Read the model definition and answer for the solid it produces. Units are mm, in the model's axes. Coordinates: 2 decimals unless noted, no trailing zeros. Write each loop counter-clockwise with the first axis right and the second up, starting at its lowest first coordinate (ties: lowest second). Pieces come first, ordered by that corner, then holes. Notation, with made-up numbers: (23.25, 56.5) -> (44.25, 56.5) arc R17 ccw to (44.25, 65.5) -> close; hole circle Ø7 at (46, -25.75). An arc over 180 degrees is marked (long way). Use CSV: the item, a comma, the result in double quotes.
Autodesk Inventor part; units mm, degrees
ref_plane "YZ Plane" through (0, 0, 0) normal (1, 0, 0) x (0, 1, 0)
ref_plane "XZ Plane" through (0, 0, 0) normal (0, 1, 0) x (-1, 0, 0)
ref_plane "XY Plane" through (0, 0, 0) normal (0, 0, 1) x (1, 0, 0)
sketch "Sketch1" plane through (0, 0, 0) normal (0, 0, 1) x (1, 0, 0)
  line L0 (0, 0) -> (5.08, 0)
  line L1 (5.08, 0) -> (5.08, 7.62)
  line L2 (0, 7.62) -> (0, 0)
  arc A0 (5.08, 7.62) -> (0, 7.62) centre (2.54, 7.62) ccw
  dimension "d0" = 5.08
  dimension "d1" = 7.62
extrude "Extrusion1" add sketch "Sketch1" along normal blind 19.05
sketch "Sketch2" plane through (5.08, 0, 0) normal (1, 0, 0) x (0, 0, -1)
  line L0 (-19.05, 7.62) -> (-19.05, 0)
  line L1 (0, 0) -> (0, 7.62)
  line L2 (0, 7.62) -> (-19.05, 7.62)
  line L3 (0, 7.62) -> (0, 10.16)
  line L4 (0, 10.16) -> (-12.7, 10.16)
  line L5 (-12.7, 10.16) -> (-19.05, 5.08)
  line L6 (-19.05, 5.08) -> (-19.05, 10.16)
  line L7 (-19.05, 10.16) -> (-12.7, 10.16)
  dimension "d4" = 12.7
  dimension "d5" = 5.08
  dimension "d6" = 2.54
extrude "Extrusion2" cut sketch "Sketch2" against normal through all contours L2 L5 L0 | L6 L7 L5 L2
properties part number "tensioning wedge"
1. A cutting plane is placed at A-A (x = 2.54). Give the vertices of the cut face in (y, z).
Solutions:
outline,"(0, 0) -> (10.16, 0) -> (10.16, 12.7) -> (5.08, 19.05) -> (0, 19.05) -> close"
2. A cutting plane is placed at B-B (z = 16.5). Give the vertices of the cut face in (x, y), and give its area (3 significant figures).
Solutions:
outline,"(0, 0) -> (5.08, 0) -> (5.08, 7.12) -> (0, 7.12) -> close"
area,"36.2 mm^2"
3. A cutting plane is placed at C-C (y = 7.25). Give the vertices of the cut face in (x, z).
Solutions:
outline,"(0, 0) -> (5.08, 0) -> (5.08, 16.34) -> (0, 16.34) -> close"
4. Find the intervals of material crossed by line 1 along Z through (x, y) = (0.75, 9); line 2 along Z through (x, y) = (2.1, 6.25); line 3 along X through (y, z) = (9.25, 3.5), in increasing order.
Solutions:
line 1,"z = 0 to 14.15"
line 2,"z = 0 to 17.59"
line 3,"x = 0.59 to 4.49"
5. A cutting plane is placed at D-D (x = 1.55). Give the vertices of the cut face in (y, z), and give its area (3 significant figures).
Solutions:
outline,"(0, 0) -> (9.96, 0) -> (9.96, 12.95) -> (5.08, 19.05) -> (0, 19.05) -> close"
area,"175 mm^2"
